Source: CAD feature listing. Evaluate the final solid. Frame: model axes, mm. A direction names the side the tool comes from. Round coordinates to 2 decimals unless told otherwise and drop trailing zeros. Write each loop counter-clockwise with the first axis right and the second up, starting at its lowest first coordinate (ties: lowest second). Pieces come first, ordered by that corner, then holes. Notation, with made-up numbers: (25.25, 49.25) -> (50.25, 49.25) arc R14 ccw to (50.25, 55.25) -> close; hole circle Ø7 at (-21, -25). An arc over 180 degrees is marked (long way). Return JSON: item names as keys, results as strings. Group by question number.
from build123d import *

# Parameters (mm, degrees)
SKETCH_1_R          = 9.4
EXTRUDE_1_DEPTH     = 15.5
SKETCH_3_R          = 6.5
EXTRUDE_2_DEPTH     = 2
SKETCH_5_R          = 10.5
EXTRUDE_4_DEPTH     = 17
SKETCH_4_R          = 4.25
CUT_EXTRUDE_1_DEPTH = 31


with BuildPart() as part:
    # 草图1 → 凸台-拉伸1 (new body)
    with BuildSketch(Plane(origin=(0, 0, 0), x_dir=(1, 0, 0), z_dir=(0, 1, 0))):
        with Locations(Location((0, 0, 0), (0, 0, 270))):
            Circle(SKETCH_1_R)
    extrude(amount=EXTRUDE_1_DEPTH)

    # 草图2 → 旋转1 (revolve)
    with BuildSketch(Plane.XY, mode=Mode.PRIVATE) as revolve_1_sk:
        Polygon((0, 18.9), (12.8, 18.9), (9.4, 15.5), (0, 15.5), align=None)
    revolve(revolve_1_sk.sketch.rotate(Axis((0, 15.5, 0), (0, 1, 0)), 270), axis=Axis((0, 15.5, 0), (0, 1, 0)))

    # 草图3 → 凸台-拉伸2 (add)
    with BuildSketch(Plane(origin=(0, 18.9, 0), x_dir=(1, 0, 0), z_dir=(0, 1, 0))):
        with Locations(Location((0, 0, 0), (0, 0, 270))):
            Circle(SKETCH_3_R)
    extrude(amount=EXTRUDE_2_DEPTH)

    # 草图5 → 凸台-拉伸4 (add)
    with BuildSketch(Plane.XZ):
        with Locations(Location((0, 0, 0), (0, 0, 270))):
            Circle(SKETCH_5_R)
    extrude(amount=-EXTRUDE_4_DEPTH)

    # 草图4 → 切除-拉伸1 (cut)
    with BuildSketch(Plane(origin=(0, 20.9, 0), x_dir=(1, 0, 0), z_dir=(0, 1, 0))):
        with Locations(Location((0, 0, 0), (0, 0, 270))):
            Circle(SKETCH_4_R)
    extrude(amount=-CUT_EXTRUDE_1_DEPTH, mode=Mode.SUBTRACT)


solid = part.part
Item 1: Cut plane D-D on y = 3.5. Output: boundary loops of the cut face in (x, z), and give its area (3 significant figures).
Item 2: First-contact query: pin 1 Ø10 at (x, y) = (-3.5, 7) entering from -Z; pin 2 Ø6 at (y, z) = (13.5, -1.5) entering from -X; pin 3 Ø6 at (x, y) = (-6.5, 7) entering from -Z. Flat tips, straight axial feed; report the tip coordinate or a pass-through.
Item 3: Cut plane A-A on x = 0. Output: boundary loops of the cut face in (y, z).
Item 4: Cut plane B-B on z = 0. Output: boundary loops of the cut face in (x, y), and give its area (3 significant figures).
Item 5: Cut plane C-C on y = 18.5. Output: boundary loops of the cut face in (x, z), and give its area (3 significant figures).
Item 6: Set-up query: faces 1 (the cylindrical face through (3.2, 8.2, -10)), 2 (the cylindrical face through (4.214, 10.596, -0.553)), 3 (the flat face through (3, 18.9, 6)). Return all of +Z, -Z, +X, -X, +Y, -Y with unobstructed straight access to the full face (end or side cutting, diameter ignored); none if empty.
Item 7: Material intervals for probe 1 along X at (y, z) = (7.25, 0); probe 2 along X at (y, z) = (15.25, 2); probe 3 along X at (y, z) = (12, 8.25), sorted ascending.
Here are the results:
{
 "1": {"outline": "circle Ø21 at (0, 0); hole circle Ø8.5 at (0, 0)", "area": "290 mm^2"},
 "2": {"pin 1": "stops at z = -10.5", "pin 2": "stops at x = -10.5", "pin 3": "stops at z = -9.9"},
 "3": {"outline": "(0, -10.5) -> (16.6, -10.5) -> (18.9, -12.8) -> (18.9, -6.5) -> (20.9, -6.5) -> (20.9, -4.25) -> (0, -4.25) -> close; (0, 4.25) -> (20.9, 4.25) -> (20.9, 6.5) -> (18.9, 6.5) -> (18.9, 12.8) -> (16.6, 10.5) -> (0, 10.5) -> close"},
 "4": {"outline": "(-12.8, 18.9) -> (-10.5, 16.6) -> (-10.5, 0) -> (-4.25, 0) -> (-4.25, 20.9) -> (-6.5, 20.9) -> (-6.5, 18.9) -> close; (4.25, 0) -> (10.5, 0) -> (10.5, 16.6) -> (12.8, 18.9) -> (6.5, 18.9) -> (6.5, 20.9) -> (4.25, 20.9) -> close", "area": "251 mm^2"},
 "5": {"outline": "circle Ø24.8 at (0, 0); hole circle Ø8.5 at (0, 0)", "area": "426 mm^2"},
 "6": {"face 1": "-Y", "face 2": "+Y, -Y", "face 3": "+Y"},
 "7": {"probe 1": "x = -10.5 to -4.25, 4.25 to 10.5", "probe 2": "x = -10.31 to -3.75, 3.75 to 10.31", "probe 3": "x = -6.5 to 6.5"}
}
